CAD build for the part. Positions are in the model's coordinates, mm. Face numbers are marked on the shaded views. A direction names the side the tool comes from. Give positions to 0.01 mm unless a question says otherwise; leave off trailing zeros. Write each loop counter-clockwise with the first axis right and the second up, starting at its lowest first coordinate (ties: lowest second). Pieces come first, ordered by that corner, then holes. Notation, with made-up numbers: (67, 20) - (117, 20) arc R25 cw to (117, 45) - close; hole circle Ø4 at (54, 58.5). An arc over 180 degrees is marked (long way). Answer as a JSON object with one key per item and string values.
from build123d import *

# Parameters (mm, degrees)
SKETCH1_W                       = 68.7568
SKETCH1_H                       = 32.004
SKETCH2_R                       = 31.877
BOSS_EXTRUDE1_DEPTH             = 8.2296
SKETCH3_R                       = 15.0368
BOSS_EXTRUDE2_DEPTH             = 5
SKETCH4_R                       = 31.877
BOSS_EXTRUDE3_DEPTH             = 8.2296
SKETCH5_R                       = 9.525
BOSS_EXTRUDE4_DEPTH             = 4
SKETCH6_R                       = 4
BOSS_EXTRUDE5_DEPTH             = 31.6
F_21_0_159_DIAMETER_HOLE1_D     = 4.0386
F_21_0_159_DIAMETER_HOLE1_DEPTH = 13.6144
F_21_0_159_DIAMETER_HOLE1_TIP   = 1.213317848
CHAMFER1_SIZE                   = 1.016
CHAMFER2_SIZE                   = 0.5
FILLET1_R                       = 1


with BuildPart() as part:
    # Sketch1 → Revolve1 (revolve)
    with BuildSketch(Plane.XY):
        with Locations((42.608, 16.002)):
            Rectangle(SKETCH1_W, SKETCH1_H)
    revolve(axis=Axis((8.2296, 0, 0), (1, 0, 0)))

    # Sketch2 → Boss-Extrude1 (add)
    with BuildSketch(Plane(origin=(76.9864, 0, 0), x_dir=(0, 0, -1), z_dir=(1, 0, 0))):
        Circle(SKETCH2_R)
    extrude(amount=BOSS_EXTRUDE1_DEPTH)

    # Sketch3 → Boss-Extrude2 (add)
    with BuildSketch(Plane(origin=(85.216, 0, 0), x_dir=(0, 0, -1), z_dir=(1, 0, 0))):
        Circle(SKETCH3_R)
    extrude(amount=BOSS_EXTRUDE2_DEPTH)

    # Sketch4 → Boss-Extrude3 (add)
    with BuildSketch(Plane.ZY.offset(-8.2296)):
        Circle(SKETCH4_R)
    extrude(amount=BOSS_EXTRUDE3_DEPTH)

    # Sketch5 → Boss-Extrude4 (add)
    with BuildSketch(Plane.ZY):
        Circle(SKETCH5_R)
    extrude(amount=BOSS_EXTRUDE4_DEPTH)

    # Sketch6 → Boss-Extrude5 (add)
    with BuildSketch(Plane.ZY.offset(4)):
        Circle(SKETCH6_R)
    extrude(amount=BOSS_EXTRUDE5_DEPTH)

    # Sketch8 → Revolve2 (revolve)
    with BuildSketch(Plane.XY.offset(-18.607090683)):
        Polygon((85.216, 15.525359639), (85.216, 11.207359639), (87.4639, 11.207359639), (87.4639, 13.325359639), (85.2639, 15.525359639), align=None)
    revolve(axis=Axis((85.216, 11.207359639, -18.607090683), (1, 0, 0)))

    # Sketch9 → Revolve3 (revolve)
    with BuildSketch(Plane.XY.offset(-11.207359639)):
        Polygon((85.216, 22.925090683), (85.216, 18.607090683), (87.4639, 18.607090683), (87.4639, 20.725090683), (85.2639, 22.925090683), align=None)
    revolve(axis=Axis((85.216, 18.607090683, -11.207359639), (1, 0, 0)))

    # #21 (0.159) Diameter Hole1
    with Locations(Plane.ZY):
        with Locations((0, 25.4), (0, -25.4)):
            Hole(F_21_0_159_DIAMETER_HOLE1_D / 2, depth=F_21_0_159_DIAMETER_HOLE1_DEPTH)
            with Locations((0, 0, -(F_21_0_159_DIAMETER_HOLE1_DEPTH + F_21_0_159_DIAMETER_HOLE1_TIP / 2))):  # 118° drill point
                Cone(0, F_21_0_159_DIAMETER_HOLE1_D / 2, F_21_0_159_DIAMETER_HOLE1_TIP, mode=Mode.SUBTRACT)

    # Chamfer1
    chamfer1_edges = [part.edges().sort_by_distance(p)[0] for p in [
        (90.216, 0, 15.0368),
        (-4, 0, -9.525),
    ]]
    chamfer(chamfer1_edges, length=CHAMFER1_SIZE)

    # Chamfer2
    chamfer2_edges = [part.edges().sort_by_distance(p)[0] for p in [
        (-35.6, 0, -4),
    ]]
    chamfer(chamfer2_edges, length=CHAMFER2_SIZE)

    # Fillet1
    fillet1_edges = [part.edges().sort_by_distance(p)[0] for p in [
        (0, 0, -31.877),
        (85.216, 0, 31.877),
    ]]
    fillet(fillet1_edges, radius=FILLET1_R)


solid = part.part
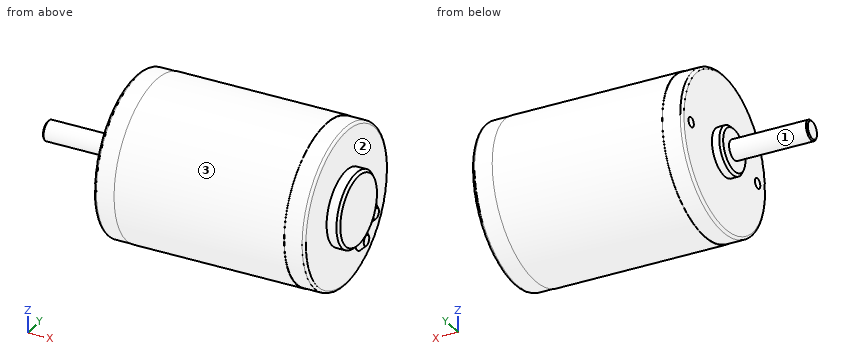
(1) Probe L1, parallel to Y at x = 5.75, z = 0; L2, parallel to Y at x = 47.5, z = -0.5; L3, parallel to X at y = -15, z = 18.5. List the from-to ranges inside material, lowest first. Write a range as [from, to].
Answer key:
{"L1": "y = [-31.88, -27.42], [-23.38, 23.38], [27.42, 31.88]", "L2": "y = [-32, 32]", "L3": "x = [0, 85.22]"}
(2) 3-axis set-ups, long thin cutter, end or side, ignore diameter. For the marked faces 1, 2 and 3: which of +Z, -Z, +X, -X, +Y, -Y reach the whole face in a straight line?
Answer key:
{"face 1": "-X", "face 2": "+X", "face 3": "+X, -X"}
(3) Saw through at C-C, the plane x = 22. Give the cut face in (y, z).
Answer key:
{"outline": "circle Ø64.01 at (0, 0)"}
(4) Flat gauge pins, fed straight in: P1, Ø12, axis at x = 19, z = -24.5, coming from the -Y side; P2, Ø6.5, axis at y = 25.4, z = 0, coming from the +X side; P3, Ø5, axis at x = -5.5, y = -7.5, coming from the +Z side; P4, Ø12, axis at y = 7, z = 4.5, coming from the -X side. Where does each tip first touch, or does it go through?
Answer key:
{"P1": "stops at y = -26.12", "P2": "stops at x = 85.22", "P3": "stops at z = 6.73", "P4": "stops at x = -35.6"}
(5) Saw through at B-B, the plane x = -13. Give the cut face in (y, z), and give its area (3 significant figures).
Answer key:
{"outline": "circle Ø8 at (0, 0)", "area": "50.3 mm²"}
